from build123d import *

# Parameters (mm, degrees)
BOSS_EXTRUDE1_DEPTH = 3
SKETCH2_W           = 3
SKETCH2_H           = 20
SKETCH2_W_2         = 40
SKETCH2_H_2         = 3
CUT_EXTRUDE2_DEPTH  = 3


with BuildPart() as part:
    # Sketch1 → Boss-Extrude1 (new body)
    with BuildSketch(Plane.XY):
        Polygon((-60, 5.09773753), (-60, -50), (-70, -50), (-70, -47), (-90, -47), (-90, -50), (-100, -50), (-100, 50), (100, 50), (100, -50), (90, -50), (90, -47), (70, -47), (70, -50), (60, -50), (60, -40.178411678), (60, 20), (-60, 20), align=None)
    extrude(amount=BOSS_EXTRUDE1_DEPTH)

    # Sketch2 → Cut-Extrude2 (cut)
    with BuildSketch(Plane.XY.offset(3)):
        Polygon((-100, 47), (-100, 30), (-97, 30), (-97, 47), (-60, 47), (-60, 50), (-100, 50), align=None)
        with Locations((-98.5, 0)):
            Rectangle(SKETCH2_W, SKETCH2_H)
        with Locations((-98.5, -40)):
            Rectangle(SKETCH2_W, SKETCH2_H)
        with Locations((0, 48.5)):
            Rectangle(SKETCH2_W_2, SKETCH2_H_2)
        Polygon((100, 50), (60, 50), (60, 47), (97, 47), (97, 30), (100, 30), (100, 47), align=None)
        with Locations((98.5, 0)):
            Rectangle(SKETCH2_W, SKETCH2_H)
        with Locations((98.5, -40)):
            Rectangle(SKETCH2_W, SKETCH2_H)
    extrude(amount=-CUT_EXTRUDE2_DEPTH, mode=Mode.SUBTRACT)


solid = part.part
Can you work these out from the model? Positions are in its coordinate system, mm. Coordinates: 2 decimals unless noted, no trailing zeros. Write each loop counter-clockwise with the first axis right and the second up, starting at its lowest first coordinate (ties: lowest second). Pieces come first, ordered by that corner, then holes. Notation, with made-up numbers: M 25,12.5 L 63,12.5 A25 ccw 63,38.5 Z; hole C -20.5,57.5 d7. An arc over 180 degrees is marked long. Use one line per item in the form item = value.
Q1. I need wall thicknesses on line 1 along X through (y, z) = (14, 0.35); line 2 along X through (y, z) = (-32, 1.9); line 3 along Y through (x, z) = (-25.5, 1.6). Which ranges of each line are inside material? Lowest first, please. Write a range as from..to.
Model answer:
line_1 = -100..-60, 60..100
line_2 = -97..-60, 60..97
line_3 = 20..50
Q2. If we section it at C-C (y = 33): Write out the boundary of the cut face in (x, z).
Model answer:
outline = M -97,0 L 97,0 L 97,3 L -97,3 Z
Q3. If we section it at A-A (y = -26): Write out the boundary of the cut face in (x, z).
Model answer:
outline = M -100,0 L -60,0 L -60,3 L -100,3 Z; M 60,0 L 100,0 L 100,3 L 60,3 Z
Q4. If we section it at D-D (y = 7.5): Write out the boundary of the cut face in (x, z), then the cut area to 3 significant figures.
Model answer:
outline = M -97,0 L -60,0 L -60,3 L -97,3 Z; M 60,0 L 97,0 L 97,3 L 60,3 Z
area = 222 mm^2
Q5. For P1, Ø1.5, axis at y = 48, z = 1.5, coming from the +X side; P2, Ø1.5, axis at x = -14.5, z = 2, coming from the +Y side; P3, Ø0.9, axis at x = 98.5, z = 2, coming from the -Y side, each with a flat end and sliding along its axis, tell me the tip position at first contact or that it passes through.
Model answer:
P1 = 60
P2 = 47
P3 = -30
Q6. If we section it at B-B (x = 6.5): Write out the boundary of the cut face in (y, z), then the cut area to 3 significant figures.
Model answer:
outline = M 20,0 L 47,0 L 47,3 L 20,3 Z
area = 81.0 mm^2
